Can you work these out from the model? Positions are in its coordinate system, mm. A direction names the side the tool comes from. Coordinates: 2 decimals unless noted, no trailing zeros. Order: outer loops, then holes, each group sorted by start corner. A loop starts at its lowest first (then second) coordinate and runs counter-clockwise, first axis right, second up. Notation, with made-up numbers: (-31.75, 48) -> (11.25, 48) arc R17 cw to (11.25, 58) -> close; hole circle Ø7 at (51, 70). An arc over 180 degrees is marked (long way). Answer in a Markdown table with one row per item.
```python
from build123d import *

# Parameters (mm, degrees)
SKETCH_1_R      = 0.6
EXTRUDE_1_DEPTH = 1.6


with BuildPart() as part:
    # 草图1 → 凸台-拉伸1 (new body)
    with BuildSketch(Plane(origin=(0, 0, 0), x_dir=(0, 0, -1), z_dir=(1, 0, 0))):
        Polygon((-6, 2), (-6, -2), (-2, -2), (-2, -9), (2, -9), (2, 2), align=None)
        with Locations((0, -7)):
            Circle(SKETCH_1_R, mode=Mode.SUBTRACT)
        with Locations((-4, 0)):
            Circle(SKETCH_1_R, mode=Mode.SUBTRACT)
        Circle(SKETCH_1_R, mode=Mode.SUBTRACT)
    extrude(amount=EXTRUDE_1_DEPTH)


solid = part.part
```
(1) Suppose I cut it at A-A (y = 0). Please give me the cut outline in (x, z), and give its area (3 significant figures).
Response values:
| item | result |
|---|---|
| outline | (0, -2) -> (1.6, -2) -> (1.6, -0.6) -> (0, -0.6) -> close; (0, 0.6) -> (1.6, 0.6) -> (1.6, 3.4) -> (0, 3.4) -> close; (0, 4.6) -> (1.6, 4.6) -> (1.6, 6) -> (0, 6) -> close |
| area | 8.96 mm2 |
(2) I need wall thicknesses on line 1 (Y direction, x = 0.8, z = 0); line 2 (Y direction, x = 1.1, z = 4); line 3 (Z direction, x = 1.4, y = -6.25). Which ranges of each line are inside material? Lowest first, please. Write a range as [from, to].
Response values:
| item | result |
|---|---|
| line 1 | [-9, -7.6], [-6.4, -0.6], [0.6, 2] |
| line 2 | [-2, -0.6], [0.6, 2] |
| line 3 | [-2, 2] |
(3) Will these pins go through, and if not, where does the flat tip stop? pin 1 Ø1.6 at (y, z) = (0, 4) entering from +X; pin 2 Ø0.5 at (x, z) = (1, 4) entering from -Y; pin 3 Ø1 at (y, z) = (0, 0) entering from -X (3 decimals); pin 4 Ø0.5 at (x, y) = (0.5, -7) entering from +Z.
Response values:
| item | result |
|---|---|
| pin 1 | x = 1.6 |
| pin 2 | y = -2 |
| pin 3 | through |
| pin 4 | z = 2 |
(4) On a 3-axis mill with a long thin cutter (end or side, diameter ignored), from which of +Z, -Z, +X, -X, +Y, -Y can I reach the whole of each face in a straight line? I mean faces 1 (the cylindrical face through (0.789, -7.586, 0.13)), 2 (the flat face through (1, -5, 2)). Say none if no direction works.
Response values:
| item | result |
|---|---|
| face 1 | +X, -X |
| face 2 | +Z, +X, -X, -Y |
(5) Suppose I cut it at C-C (x = 1.4). Please give me the cut outline in (y, z).
Response values:
| item | result |
|---|---|
| outline | (-9, -2) -> (2, -2) -> (2, 6) -> (-2, 6) -> (-2, 2) -> (-9, 2) -> close; hole circle Ø1.2 at (-7, 0); hole circle Ø1.2 at (0, 0); hole circle Ø1.2 at (0, 4) |
(6) Suppose I cut it at B-B (z = 4). Please give me the cut outline in (x, y), and give its area (3 significant figures).
Response values:
| item | result |
|---|---|
| outline | (0, -2) -> (1.6, -2) -> (1.6, -0.6) -> (0, -0.6) -> close; (0, 0.6) -> (1.6, 0.6) -> (1.6, 2) -> (0, 2) -> close |
| area | 4.48 mm2 |
